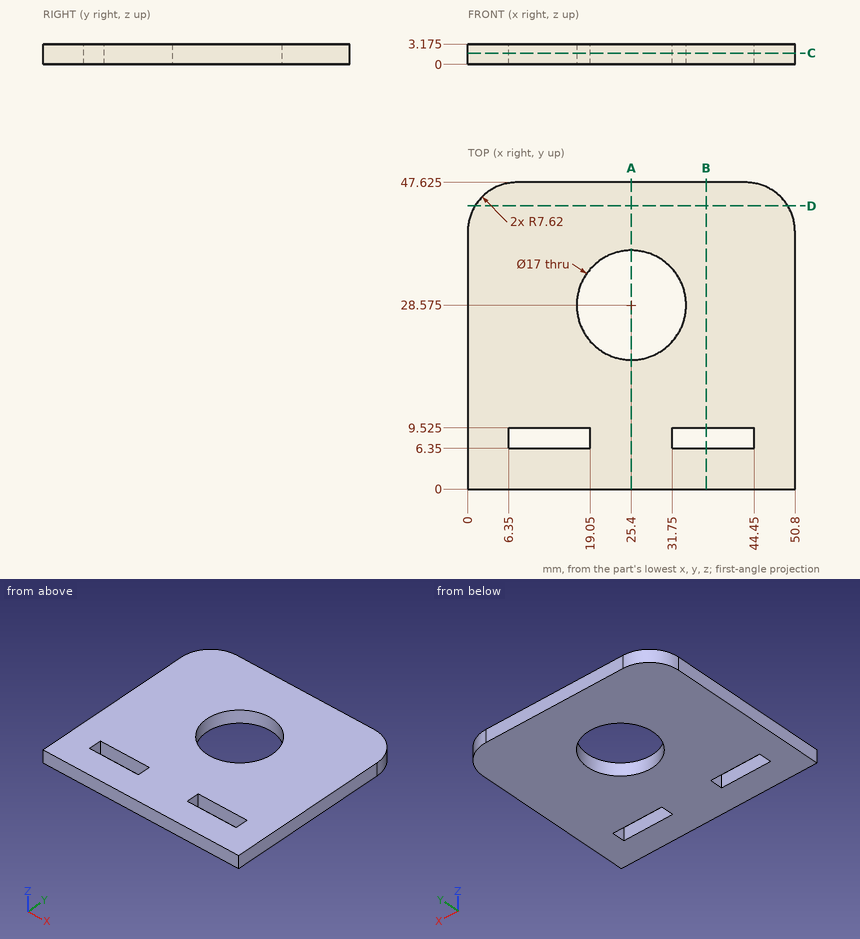
Study the drawing (mm; zero at the part's minimum x, y, z) and answer. Round coordinates to 2 decimals unless told otherwise and drop trailing zeros. Write each loop counter-clockwise with the first axis right and the second up, starting at its lowest first coordinate (ties: lowest second). Pieces come first, ordered by that corner, then holes.
1) Straight lines are drawn through the part: line 1 (X direction, y = 8, z = 2.1); line 2 (Y direction, x = 13, z = 0.5) (3 decimals); line 3 (Y direction, x = 25.4, z = 1.1) (3 decimals). For each, find the intervals that lie inside material, in ascending order.
2) A cutting plane is placed at D-D (y = 44). Give the vertices of the cut face in (x, z) (3 decimals).
3) A cutting plane is placed at A-A (x = 25.4). Give the vertices of the cut face in (y, z) (3 decimals), plus the area to 3 significant figures.
4) A cutting plane is placed at C-C (z = 1.75). Give the vertices of the cut face in (x, y) (3 decimals).
5) A cutting plane is placed at B-B (x = 37). Give the vertices of the cut face in (y, z) (3 decimals).
Completed:
1. line 1: x = 0 to 6.35, 19.05 to 31.75, 44.45 to 50.8
1. line 2: y = 0 to 6.35, 9.525 to 47.625
1. line 3: y = 0 to 20.075, 37.075 to 47.625
2. outline: (1.131, 0) - (49.669, 0) - (49.669, 3.175) - (1.131, 3.175) - close
3. outline: (0, 0) - (20.075, 0) - (20.075, 3.175) - (0, 3.175) - close; (37.075, 0) - (47.625, 0) - (47.625, 3.175) - (37.075, 3.175) - close
3. area: 97.2 mm2
4. outline: (0, 0) - (50.8, 0) - (50.8, 40.005) arc R7.62 ccw to (43.18, 47.625) - (7.62, 47.625) arc R7.62 ccw to (0, 40.005) - close; hole (6.35, 6.35) - (19.05, 6.35) - (19.05, 9.525) - (6.35, 9.525) - close; hole circle Ø17 at (25.4, 28.575); hole (31.75, 6.35) - (44.45, 6.35) - (44.45, 9.525) - (31.75, 9.525) - close
5. outline: (0, 0) - (6.35, 0) - (6.35, 3.175) - (0, 3.175) - close; (9.525, 0) - (47.625, 0) - (47.625, 3.175) - (9.525, 3.175) - close
